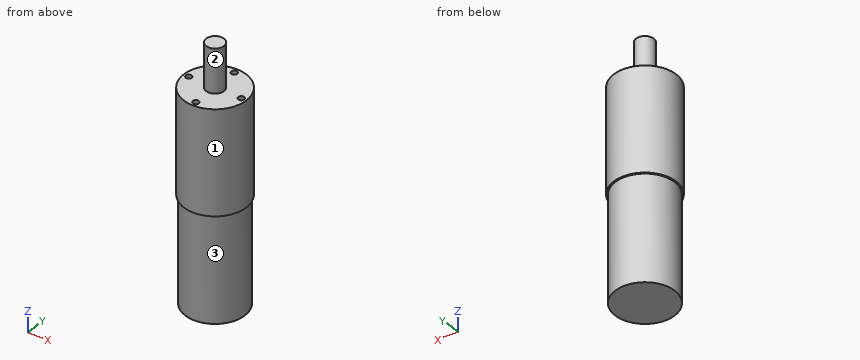
```python
from build123d import *

# Parameters (mm, degrees)
SZKIC1_R                    = 21
DODANIE_WYCI_GNI_CIE1_DEPTH = 70
SZKIC2_R                    = 2
WYTNIJ_WYCI_GNI_CIE1_DEPTH  = 6
SZKIC3_R                    = 6
DODANIE_WYCI_GNI_CIE2_DEPTH = 29.5
SZKIC4_R                    = 20
DODANIE_WYCI_GNI_CIE3_DEPTH = 71


with BuildPart() as part:
    # Szkic1 → Dodanie-wyciągnięcie1 (new body)
    with BuildSketch(Plane.XY):
        Circle(SZKIC1_R)
    extrude(amount=DODANIE_WYCI_GNI_CIE1_DEPTH)

    # Szkic2 → Wytnij-wyciągnięcie1 (cut)
    with BuildSketch(Plane.XY.offset(70)):
        with Locations((0, 17.5)):
            Circle(SZKIC2_R)
        with Locations((17.5, 0)):
            Circle(SZKIC2_R)
        with Locations((0, -17.5)):
            Circle(SZKIC2_R)
        with Locations((-17.5, 0)):
            Circle(SZKIC2_R)
    extrude(amount=-WYTNIJ_WYCI_GNI_CIE1_DEPTH, mode=Mode.SUBTRACT)

    # Szkic3 → Dodanie-wyciągnięcie2 (add)
    with BuildSketch(Plane.XY.offset(70)):
        Circle(SZKIC3_R)
    extrude(amount=DODANIE_WYCI_GNI_CIE2_DEPTH)

    # Szkic4 → Dodanie-wyciągnięcie3 (add)
    with BuildSketch(Plane(origin=(0, 0, 0), x_dir=(-1, 0, 0), z_dir=(0, 0, -1))):
        Circle(SZKIC4_R)
    extrude(amount=DODANIE_WYCI_GNI_CIE3_DEPTH)


solid = part.part
```
Input: part model. Units: mm. Frame: model coordinates. Face numbers are marked on the shaded views. A direction names the side the tool comes from. Coordinates: 2 decimals unless noted, no trailing zeros. Order: outer loops, then holes, each group sorted by start corner. A loop starts at its lowest first (then second) coordinate and runs counter-clockwise, first axis right, second up. Notation, with made-up numbers: (72, 46.5) - (115, 46.5) arc R18 cw to (115, 74.5) - close; hole circle Ø8 at (72.5, 5). An arc over 180 degrees is marked (long way). Return JSON: item names as keys, results as strings.
Q1. Access query for the marked faces 1, 2 and 3. Directions: +Z, -Z, +X, -X, +Y, -Y. A direction counts if a zero-diameter tool reaches every point of the face in a straight line with its end or side. Return the directions, or none.
The answers:
{"face 1": "+Z, -Z", "face 2": "+Z", "face 3": "-Z"}
Q2. Cut plane D-D (y = -17.5). Return loops of the section in (x, z), then the cut area to 3 significant figures.
The answers:
{"outline": "(-11.61, 0) - (-9.68, 0) - (-9.68, -71) - (9.68, -71) - (9.68, 0) - (11.61, 0) - (11.61, 70) - (2, 70) - (2, 64) - (-2, 64) - (-2, 70) - (-11.61, 70) - close", "area": "2,980 mm2"}
Q3. First-contact query: pin 1 (10 mm diameter, centred on y = 6, z = 43, fed in from +X); pin 2 (10 mm diameter, centred on x = -16, z = 32, fed in from -Y); pin 3 (2 mm diameter, centred on x = -9.5, y = -15.5, fed in from +Z). Flat tips, straight axial feed; report the tip coordinate or a pass-through.
The answers:
{"pin 1": "stops at x = 20.98", "pin 2": "stops at y = -17.89", "pin 3": "stops at z = 70"}
Q4. Cut plane C-C (z = 31). Return loops of the section in (x, y), then the cut area to 3 significant figures.
The answers:
{"outline": "circle Ø42 at (0, 0)", "area": "1,390 mm2"}
Q5. Cut plane A-A (x = 0). Return loops of the section in (y, z).
The answers:
{"outline": "(-21, 0) - (-20, 0) - (-20, -71) - (20, -71) - (20, 0) - (21, 0) - (21, 70) - (19.5, 70) - (19.5, 64) - (15.5, 64) - (15.5, 70) - (6, 70) - (6, 99.5) - (-6, 99.5) - (-6, 70) - (-15.5, 70) - (-15.5, 64) - (-19.5, 64) - (-19.5, 70) - (-21, 70) - close"}
Q6. Ray query, probe 1 along Y at (x, z) = (0, 66.05); probe 2 along Y at (x, z) = (1, -31); probe 3 along X at (y, z) = (17, 66). Return the intervals inside material, ascending.
The answers:
{"probe 1": "y = -21 to -19.5, -15.5 to 15.5, 19.5 to 21", "probe 2": "y = -19.97 to 19.97", "probe 3": "x = -12.33 to -1.94, 1.94 to 12.33"}
